```python
from build123d import *

# Parameters (mm, degrees)
F0_R     = 12.7
F1_DEPTH = 152.4
F2_R     = 38.1
F3_DEPTH = 42.949663
F5_DEPTH = 152.401
F6_W     = 157.67442
F6_H     = 101.6
F7_DEPTH = 838.2


with BuildPart() as f1:
    # F0 (on Top) → F1 (new body)
    with BuildSketch(Plane.XY):
        with BuildLine():
            ThreePointArc((87.912252, -17.548663), (115.728859, -23.575235), (131.675379, 0))
            ThreePointArc((131.675379, 0), (113.700373, 24.290522), (85.216366, 14.201337))
            ThreePointArc((85.216366, 14.201337), (80.96645, -2.148976), (87.912252, -17.548663))
        make_face()
        with Locations((106.275379, 0)):
            Circle(F0_R, mode=Mode.SUBTRACT)
        with BuildLine():
            ThreePointArc((87.912252, -17.548663), (80.96645, -2.148976), (85.216366, 14.201337))
            Line((85.216366, 14.201337), (-96.924621, 14.201337))
            Line((-96.924621, 14.201337), (-96.924621, -17.548663))
            Line((-96.924621, -17.548663), (87.912252, -17.548663))
        make_face()
    extrude(amount=F1_DEPTH)

    # F2 (on face) → F3 (cut, through all)
    with BuildSketch(Plane.XZ.offset(17.548663)):
        with BuildLine():
            ThreePointArc((-96.924621, 76.2), (-74.606158, 130.081537), (-20.724621, 152.4))
            Line((-20.724621, 152.4), (-96.924621, 152.4))
            Line((-96.924621, 152.4), (-96.924621, 76.2))
        make_face()
        with BuildLine():
            ThreePointArc((-20.724621, 0), (-74.606158, 22.318463), (-96.924621, 76.2))
            Line((-96.924621, 76.2), (-96.924621, 0))
            Line((-96.924621, 0), (-20.724621, 0))
        make_face()
        Polygon((-96.924621, 0), (-96.924621, 76.2), (-96.924621, 152.4), (-108.673256, 152.4), (-108.673256, 0), align=None)
        with Locations((-20.724621, 76.2)):
            Circle(F2_R)
    extrude(amount=-F3_DEPTH, mode=Mode.SUBTRACT)

    # F4 (on face) → F5 (cut, through all)
    with BuildSketch(Plane.XY.offset(152.4)):
        with BuildLine():
            Line((-8.024621, -8.023663), (42.775379, -8.023663))
            ThreePointArc((42.775379, -8.023663), (49.125379, -1.673663), (42.775379, 4.676337))
            Line((42.775379, 4.676337), (-8.024621, 4.676337))
            ThreePointArc((-8.024621, 4.676337), (-14.374621, -1.673663), (-8.024621, -8.023663))
        make_face()
    extrude(amount=-F5_DEPTH, mode=Mode.SUBTRACT)

    # F6 (on face) → F7 (cut, symmetric)
    with BuildSketch(Plane.XZ.offset(17.548663)):
        with Locations((147.012589, 76.2)):
            Rectangle(F6_W, F6_H)
    extrude(amount=F7_DEPTH, both=True, mode=Mode.SUBTRACT)


solid = f1.part
```
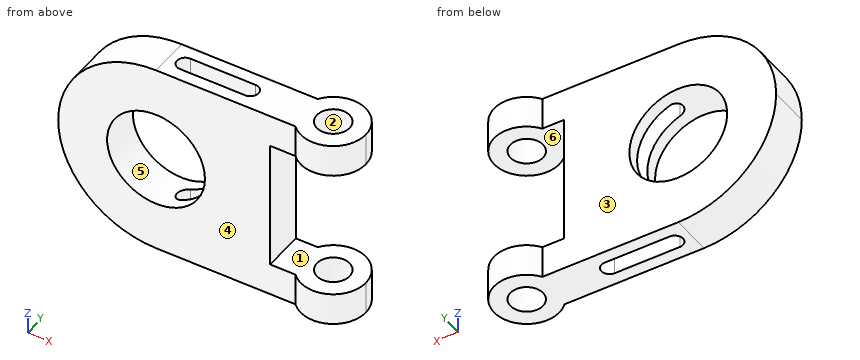
Build history of the part. All positions in model axes, mm. Face numbers are marked on the shaded views. A direction names the side the tool comes from. Give positions to 0.01 mm unless a question says otherwise; leave off trailing zeros. Loops run counter-clockwise (first coordinate to the right, second up) from the corner with the lowest first, then second, coordinate; pieces in that order, holes last. Notation, with made-up numbers: (42, 9) -> (62, 9) arc R18 ccw to (62, 37) -> close; hole circle Ø2 at (81.25, 58.25). An arc over 180 degrees is marked (long way). One line per question, with ' | ' between items.
Q1. Cut at B-B, the plane z = 53. Write the cut outline in (x, y), plus the area to 3 significant figures.
Filled sheet:
outline: (-93.31, -17.55) -> (-50.95, -17.55) -> (-50.95, 14.2) -> (-93.31, 14.2) -> close; (9.5, -17.55) -> (68.18, -17.55) -> (68.18, 14.2) -> (9.5, 14.2) -> (9.5, 4.68) -> (42.78, 4.68) arc R6.35 cw to (42.78, -8.02) -> (9.5, -8.02) -> close | area: 2,720 mm²
Q2. Cut at A-A, the plane x = 36. Write the cut outline in (y, z), plus the area to 3 significant figures.
Filled sheet:
outline: (-17.55, 0) -> (-8.02, 0) -> (-8.02, 152.4) -> (-17.55, 152.4) -> close; (4.68, 0) -> (14.2, 0) -> (14.2, 152.4) -> (4.68, 152.4) -> close | area: 2,900 mm²
Q3. Cut at C-C, the plane x = 113. Write the cut outline in (y, z), plus the area to 3 significant figures.
Filled sheet:
outline: (-24.49, 0) -> (-10.77, 0) -> (-10.77, 25.4) -> (-24.49, 25.4) -> close; (-24.49, 127) -> (-10.77, 127) -> (-10.77, 152.4) -> (-24.49, 152.4) -> close; (10.77, 0) -> (24.49, 0) -> (24.49, 25.4) -> (10.77, 25.4) -> close; (10.77, 127) -> (24.49, 127) -> (24.49, 152.4) -> (10.77, 152.4) -> close | area: 1,390 mm²
Q4. Pull direction Y, two halves, no side cores. Call the marked faces 1, 2 and 3: pulls with the +Y half, pulls with the -Y half, needs draft (parallel to the pull), parting line crosses it, or undercut.
Filled sheet:
face 1: needs draft | face 2: undercut | face 3: pulls with the +Y half
Q5. Cut at D-D, the plane z = 137. Write the cut outline in (x, y), plus the area to 3 significant figures.
Filled sheet:
outline: (-66.66, -17.55) -> (87.91, -17.55) arc R25.4 ccw (long way) to (85.22, 14.2) -> (-66.66, 14.2) -> close; hole (-8.02, -8.02) -> (42.78, -8.02) arc R6.35 ccw to (42.78, 4.68) -> (-8.02, 4.68) arc R6.35 ccw to start; hole circle Ø25.4 at (106.28, 0) | area: 5,490 mm²
Q6. Drop flat-ended pins along their axis: pin 1 (15 mm diameter, centred on x = 107, y = 4, fed in from -Z); pin 2 (1 mm diameter, centred on x = -60, y = 1.5, fed in from +Z); pin 3 (15 mm diameter, centred on x = 27.5, z = 67.5, fed in from -Y); pin 4 (8 mm diameter, centred on y = -1.5, z = 101.5, fed in from +X). Give the stop position or say it passes through.
Filled sheet:
pin 1: passes through | pin 2: stops at z = 141.8 | pin 3: stops at y = -17.55 | pin 4: stops at x = 68.18
Q7. Tool access for the marked faces 4, 5 and 6: list every direction of +Z, -Z, +X, -X, +Y, -Y with a clear straight run to the whole face (end or side of a thin tool).
Filled sheet:
face 4: +Z, -Z, -X, -Y | face 5: +Y, -Y | face 6: +X, +Y, -Y
Q8. Drill centre lines: line 1 along Z through (x, y) = (107.5, -17); line 2 along Y through (x, z) = (28.5, 98); line 3 along X through (y, z) = (4, 145). Where is each one in solid material? Low to high. Write a range as [from, to].
Filled sheet:
line 1: z = [0, 25.4], [127, 152.4] | line 2: y = [-17.55, -8.02], [4.68, 14.2] | line 3: x = [-53.48, -10.88], [45.63, 94.22], [118.33, 131.36]
